Autodesk Inventor part; units mm, degrees
ref_plane "작업 평면3" through (0, 2.2, 0) normal (0, -1, 0) x (1, 0, 0)
ref_plane "YZ Plane" through (0, 0, 0) normal (1, 0, 0) x (0, 1, 0)
ref_plane "XZ Plane" through (0, 0, 0) normal (0, 1, 0) x (-1, 0, 0)
sketch "스케치1" plane through (0, 0, 0) normal (0, 1, 0) x (-1, 0, 0)
  line L0 (-16.2959, 6.75) -> (-6.75, 16.2959)
  line L1 (-6.75, 16.2959) -> (6.75, 16.2959)
  line L2 (6.75, 16.2959) -> (16.2959, 6.75)
  line L3 (16.2959, 6.75) -> (16.2959, -6.75)
  line L4 (16.2959, -6.75) -> (6.75, -16.2959)
  line L5 (6.75, -16.2959) -> (-6.75, -16.2959)
  line L6 (-6.75, -16.2959) -> (-16.2959, -6.75)
  line L7 (-16.2959, -6.75) -> (-16.2959, 6.75)
  line L8 (19.4959, 8.0755) -> (19.4959, -8.0755)
  line L9 (19.4959, -8.0755) -> (8.0755, -19.4959)
  line L10 (8.0755, -19.4959) -> (-8.0755, -19.4959)
  line L11 (-8.0755, -19.4959) -> (-19.4959, -8.0755)
  line L12 (-19.4959, -8.0755) -> (-19.4959, 8.0755)
  line L13 (-19.4959, 8.0755) -> (-8.0755, 19.4959)
  line L14 (-8.0755, 19.4959) -> (8.0755, 19.4959)
  line L15 (8.0755, 19.4959) -> (19.4959, 8.0755)
  point P0 (0, 0)
  point P1 (0, 0)
  point P2 (0, 0)
  dimension "d0" = 13.5
  dimension "d1" = 3.2
extrude "돌출1" add sketch "스케치1" along normal blind 4.4 contours L0 L1 L2 L3 L4 L5 L6 L7 | L8 L9 L10 L11 L12 L13 L14 L15
sketch "스케치14" plane through (0, 4.4, 0) normal (0, 1, 0) x (1, 0, 0)
  line L0 (6.5843, -15.8959) -> (-6.5843, -15.8959)
  line L1 (-6.5843, -15.8959) -> (-15.8959, -6.5843)
  line L2 (-15.8959, -6.5843) -> (-15.8959, 6.5843)
  line L3 (-15.8959, 6.5843) -> (-6.5843, 15.8959)
  line L4 (-6.5843, 15.8959) -> (6.5843, 15.8959)
  line L5 (6.5843, 15.8959) -> (15.8959, 6.5843)
  line L6 (15.8959, 6.5843) -> (15.8959, -6.5843)
  line L7 (15.8959, -6.5843) -> (6.5843, -15.8959)
  line L8 (-7.4127, 17.8959) -> (7.4127, 17.8959)
  line L9 (7.4127, 17.8959) -> (17.8959, 7.4127)
  line L10 (17.8959, 7.4127) -> (17.8959, -7.4127)
  line L11 (17.8959, -7.4127) -> (7.4127, -17.8959)
  line L12 (7.4127, -17.8959) -> (-7.4127, -17.8959)
  line L13 (-7.4127, -17.8959) -> (-17.8959, -7.4127)
  line L14 (-17.8959, -7.4127) -> (-17.8959, 7.4127)
  line L15 (-17.8959, 7.4127) -> (-7.4127, 17.8959)
  line L16 (19.4959, -8.0755) -> (19.4959, 8.0755)
  point P0 (0, 0)
  point P1 (0, 0)
  point P2 (0, 0)
  dimension "d138" = 2
  dimension "d139" = 1.6
extrude "돌출16" cut sketch "스케치14" against normal blind 1.2
sketch "스케치15" plane through (0, 4.4, 0) normal (0, 1, 0) x (1, 0, 0)
  line L0 (-15.8959, -6.5843) -> (-6.5843, -15.8959)
  line L1 (-6.5843, -15.8959) -> (6.5843, -15.8959)
  line L2 (6.5843, -15.8959) -> (15.8959, -6.5843)
  line L3 (15.8959, -6.5843) -> (15.8959, 6.5843)
  line L4 (15.8959, 6.5843) -> (6.5843, 15.8959)
  line L5 (6.5843, 15.8959) -> (-6.5843, 15.8959)
  line L6 (-6.5843, 15.8959) -> (-15.8959, 6.5843)
  line L7 (-15.8959, 6.5843) -> (-15.8959, -6.5843)
  point P0 (0, 0)
extrude "돌출17" cut sketch "스케치15" against normal blind 0.6
sketch "스케치16" plane through (0, 3.8, 0) normal (0, 1, 0) x (1, 0, 0)
  line L0 (-6.0873, 14.6959) -> (6.0873, 14.6959)
  line L1 (6.0873, 14.6959) -> (14.6959, 6.0873)
  line L2 (14.6959, 6.0873) -> (14.6959, -6.0873)
  line L3 (14.6959, -6.0873) -> (6.0873, -14.6959)
  line L4 (6.0873, -14.6959) -> (-6.0873, -14.6959)
  line L5 (-6.0873, -14.6959) -> (-14.6959, -6.0873)
  line L6 (-14.6959, -6.0873) -> (-14.6959, 6.0873)
  line L7 (-14.6959, 6.0873) -> (-6.0873, 14.6959)
  line L8 (15.8959, 6.5843) -> (15.8959, -6.5843)
  point P0 (0, 0)
  point P1 (0, 0)
  dimension "d144" = 1.2
extrude "돌출18" cut sketch "스케치16" against normal up to surface (3.8 mm away)
fillet "모깎기2" radius 1.2 16 edges at (0, 4.4, -19.4959) (-13.7857, 4.4, -13.7857) (13.7857, 4.4, -13.7857) (19.4959, 4.4, 0) (13.7857, 4.4, 13.7857) (0, 4.4, 19.4959) (-13.7857, 4.4, 13.7857) (-19.4959, 4.4, 0) (-19.4959, 0, 0) (-13.7857, 0, 13.7857) (0, 0, 19.4959) (13.7857, 0, 13.7857) (-13.7857, 0, -13.7857) (0, 0, -19.4959) (19.4959, 0, 0) (13.7857, 0, -13.7857)
ref_plane "작업 평면3" through (0, 2.2, 0) normal (0, -1, 0) x (1, 0, 0)
mirror "미러6" about plane through (0, 2.2, 0) normal (0, -1, 0) of "돌출17", "돌출16"
properties part number "OV-PAM_ring_2"
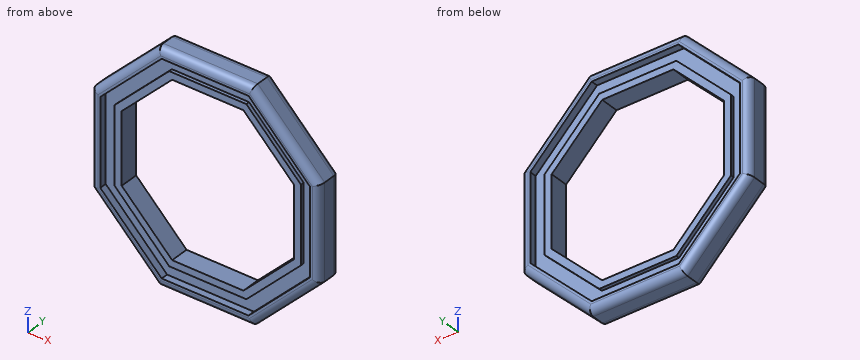
For this review, take the finished solid that the model builds, in its own axes (mm). Round coordinates to 2 decimals unless told otherwise and drop trailing zeros. Loops run counter-clockwise (first coordinate to the right, second up) from the corner with the lowest first, then second, coordinate; pieces in that order, holes last.
(1) We need section A-A (x = 3). Give the boundary of the cut face in (y, z).
Returned:
outline: (0, -18.3) arc R1.2 ccw to (1.2, -19.5) - (3.2, -19.5) arc R1.2 ccw to (4.4, -18.3) - (4.4, -17.9) - (3.2, -17.9) - (3.2, -15.9) - (3.8, -15.9) - (3.8, -14.7) - (0.6, -14.7) - (0.6, -15.9) - (1.2, -15.9) - (1.2, -17.9) - (0, -17.9) - close; (0, 17.9) - (1.2, 17.9) - (1.2, 15.9) - (0.6, 15.9) - (0.6, 14.7) - (3.8, 14.7) - (3.8, 15.9) - (3.2, 15.9) - (3.2, 17.9) - (4.4, 17.9) - (4.4, 18.3) arc R1.2 ccw to (3.2, 19.5) - (1.2, 19.5) arc R1.2 ccw to (0, 18.3) - close
(2) Clearance check with flat-ended pins moving along their axes: P1, Ø0.6, axis at x = 0.5, y = 0.5, coming from the -Z side; P2, Ø3, axis at x = -14, z = -9, coming from the +Y side; P3, Ø0.6, axis at y = 0.5, z = 3.5, coming from the +X side. State where each tip first meets the part, or that it passes through.
Returned:
P1: stops at z = -19.43
P2: stops at y = 3.8
P3: stops at x = 19.43
(3) We need section B-B (z = -1). Give the boundary of the cut face in (x, y).
Returned:
outline: (-19.5, 1.2) arc R1.2 ccw to (-18.3, 0) - (-17.9, 0) - (-17.9, 1.2) - (-15.9, 1.2) - (-15.9, 0.6) - (-14.7, 0.6) - (-14.7, 3.8) - (-15.9, 3.8) - (-15.9, 3.2) - (-17.9, 3.2) - (-17.9, 4.4) - (-18.3, 4.4) arc R1.2 ccw to (-19.5, 3.2) - close; (14.7, 0.6) - (15.9, 0.6) - (15.9, 1.2) - (17.9, 1.2) - (17.9, 0) - (18.3, 0) arc R1.2 ccw to (19.5, 1.2) - (19.5, 3.2) arc R1.2 ccw to (18.3, 4.4) - (17.9, 4.4) - (17.9, 3.2) - (15.9, 3.2) - (15.9, 3.8) - (14.7, 3.8) - close
(4) Wall thickness on line 1 along X through (y, z) = (1.25, -3); line 2 along X through (y, z) = (0.7, -5.5); line 3 along Z through (x, y) = (-3, 3.55): over which ranges is each line inside the solid? List them lowest first.
Returned:
line 1: x = -19.5 to -14.7, 14.7 to 19.5
line 2: x = -19.39 to -17.9, -15.9 to -14.7, 14.7 to 15.9, 17.9 to 19.39
line 3: z = -19.44 to -17.9, -15.9 to -14.7, 14.7 to 15.9, 17.9 to 19.44
(5) We need section C-C (y = 2.45). Give the boundary of the cut face in (x, z), plus the area to 3 significant figures.
Returned:
outline: (-19.5, -8.08) - (-8.08, -19.5) - (8.08, -19.5) - (19.5, -8.08) - (19.5, 8.08) - (8.08, 19.5) - (-8.08, 19.5) - (-19.5, 8.08) - close; hole (-14.7, -6.09) - (-6.09, -14.7) - (6.09, -14.7) - (14.7, -6.09) - (14.7, 6.09) - (6.09, 14.7) - (-6.09, 14.7) - (-14.7, 6.09) - close
area: 544 mm2
